Study the drawing (mm; zero at the part's minimum x, y, z) and answer. Give positions to 0.01 mm unless a question says otherwise; leave off trailing zeros. Order: outer loops, then holes, each group sorted by start corner. A loop starts at its lowest first (then second) coordinate and runs counter-clockwise, first axis right, second up. Notation, with made-up numbers: (-22, -14.75) -> (-2, -14.75) arc R22 ccw to (-2, -2.75) -> close; hole circle Ø3 at (40.5, -27). An arc over 180 degrees is marked (long way). Answer as CSV lines item,"result". Start each with the question number.
1. A cutting plane is placed at B-B (y = 194.5). Give the vertices of the cut face in (x, z), then the cut area to 3 significant figures.
2. Flat-ended cylindrical pins translate along their axes: pin 1 (3 mm diameter, centred on x = 4, z = 288.5, fed in from +Y); pin 2 (1.7 mm diameter, centred on x = 1.5, z = 2, fed in from -Y); pin 3 (6.5 mm diameter, centred on y = 27.98, z = 40.79, fed in from +X); pin 4 (3 mm diameter, centred on x = 1.5, y = 12.5, fed in from +Z). Find the tip coordinate at first contact, or state that the pin passes through.
3. A cutting plane is placed at A-A (x = 4.55). Give the vertices of the cut face in (y, z), then the cut area to 3 significant figures.
4. Find the intervals of material crossed by L1, parallel to Z at x = 4.05, y = 21; L2, parallel to Z at x = 5.3, y = 29.5; L3, parallel to Z at x = 1.45, y = 30 (1 decimal), in increasing order.
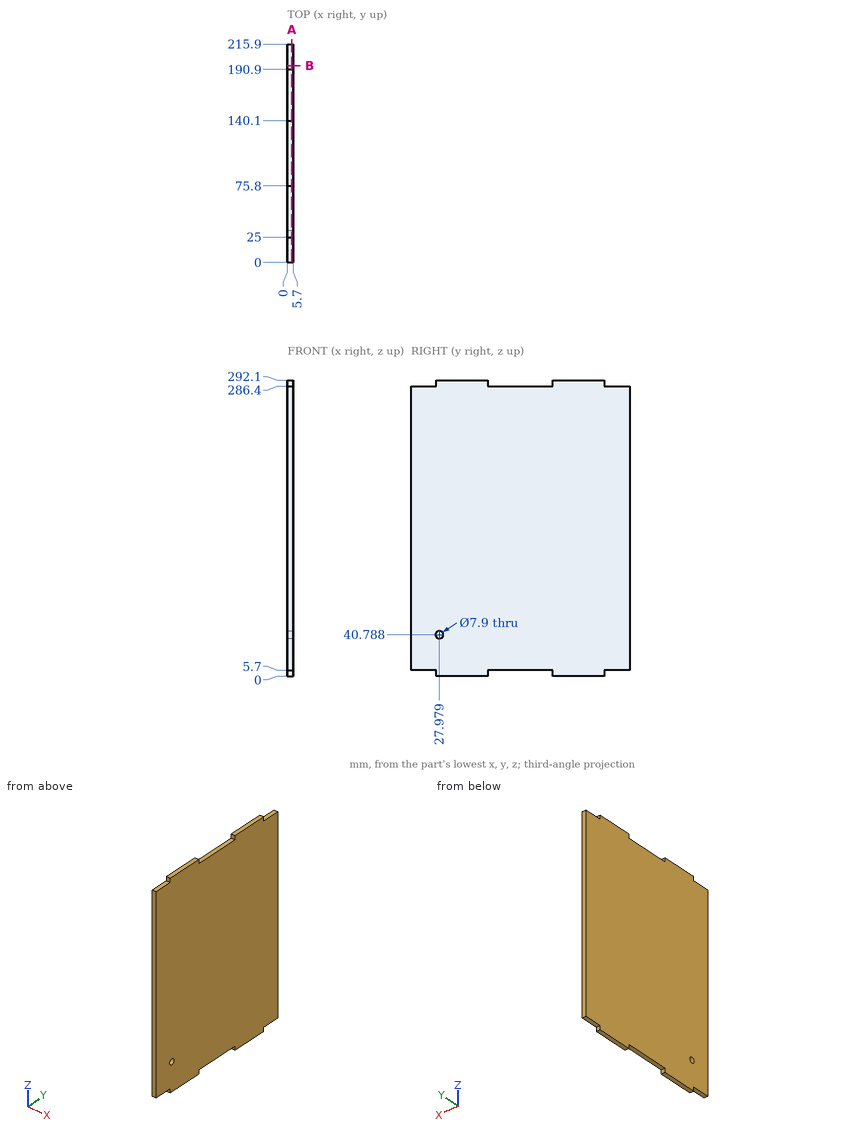
Answer sheet:
1,outline,"(0, 5.7) -> (5.7, 5.7) -> (5.7, 286.4) -> (0, 286.4) -> close"
1,area,"1,600 mm^2"
2,pin 1,"stops at y = 190.9"
2,pin 2,"stops at y = 25"
2,pin 3,"passes through"
2,pin 4,"stops at z = 286.4"
3,outline,"(0, 5.7) -> (25, 5.7) -> (25, 0) -> (75.8, 0) -> (75.8, 5.7) -> (140.1, 5.7) -> (140.1, 0) -> (190.9, 0) -> (190.9, 5.7) -> (215.9, 5.7) -> (215.9, 286.4) -> (190.9, 286.4) -> (190.9, 292.1) -> (140.1, 292.1) -> (140.1, 286.4) -> (75.8, 286.4) -> (75.8, 292.1) -> (25, 292.1) -> (25, 286.4) -> (0, 286.4) -> close; hole circle Ø7.9 at (27.98, 40.79)"
3,area,"61,700 mm^2"
4,L1,"z = 5.7 to 286.4"
4,L2,"z = 0 to 37.14, 44.43 to 292.1"
4,L3,"z = 0 to 37.4, 44.2 to 292.1"
